from build123d import *

# Parameters (mm, degrees)
F0_R     = 73.025
F1_DEPTH = 3.81
F2_R     = 73.025
F2_R_2   = 69.977
F3_DEPTH = 25.4
F4_R     = 61.2936559159
F5_DEPTH = 25.4
F7_DEPTH = 3.81
F8_W     = 59.7810531035
F8_H     = 29.3873213232
F8_W_2   = 61.7938893847
F9_DEPTH = 127


with BuildPart() as f1:
    # F0 (on Top) → F1 (new body)
    with BuildSketch(Plane.XY):
        Circle(F0_R)
    extrude(amount=F1_DEPTH)

    # F2 (on face) → F3 (join)
    with BuildSketch(Plane.XY.offset(3.81)):
        Circle(F2_R)
        Circle(F2_R_2, mode=Mode.SUBTRACT)
    extrude(amount=F3_DEPTH)

    # F4 (on face) → F5 (cut)
    with BuildSketch(Plane.XY.offset(3.81)):
        Circle(F4_R)
    extrude(amount=-F5_DEPTH, mode=Mode.SUBTRACT)

    # F6 (on face) → F7 (join, through all)
    with BuildSketch(Plane.XY.offset(3.81)):
        with BuildLine():
            Line((3.1198861543, 65.2156993747), (-3.1198873185, 65.2156993747))
            Line((-3.1198873185, 65.2156993747), (-3.1198873185, 9.1467575412))
            ThreePointArc((-3.1198873185, 9.1467575412), (-6.15e-07, 9.6642056268), (3.1198861543, 9.1467579383))
            Line((3.1198861543, 9.1467579383), (3.1198861543, 65.2156993747))
        make_face()
        with BuildLine():
            ThreePointArc((3.1198861543, 9.1467579383), (-6.15e-07, 9.6642056268), (-3.1198873185, 9.1467575412))
            Line((-3.1198873185, 9.1467575412), (-3.1198873185, 3.8243774325))
            Line((-3.1198873185, 3.8243774325), (3.1198861543, 3.8243774325))
            Line((3.1198861543, 3.8243774325), (3.1198861543, 9.1467579383))
        make_face()
        with BuildLine():
            Line((-3.1198873185, 3.8243774325), (-3.1198873185, 9.1467575412))
            ThreePointArc((-3.1198873185, 9.1467575412), (-6.5614847143, 7.0953357033), (-8.8753032428, 3.8243774325))
            Line((-8.8753032428, 3.8243774325), (-3.1198873185, 3.8243774325))
        make_face()
        with BuildLine():
            ThreePointArc((8.8753032428, 3.8243774325), (6.5614842628, 7.0953361208), (3.1198861543, 9.1467579383))
            Line((3.1198861543, 9.1467579383), (3.1198861543, 3.8243774325))
            Line((3.1198861543, 3.8243774325), (8.8753032428, 3.8243774325))
        make_face()
        with BuildLine():
            Line((-3.1198873185, -2.8179625515), (-3.1198873185, 3.8243774325))
            Line((-3.1198873185, 3.8243774325), (-8.8753032428, 3.8243774325))
            ThreePointArc((-8.8753032428, 3.8243774325), (-9.6493328393, 0.5359534999), (-9.2442391497, -2.8179625515))
            Line((-9.2442391497, -2.8179625515), (-3.1198873185, -2.8179625515))
        make_face()
        with BuildLine():
            ThreePointArc((-9.2442391497, -2.8179625515), (-9.6493328393, 0.5359534999), (-8.8753032428, 3.8243774325))
            Line((-8.8753032428, 3.8243774325), (-63.3035078645, 3.8243774325))
            Line((-63.3035078645, 3.8243774325), (-63.3035078645, -2.8179625515))
            Line((-63.3035078645, -2.8179625515), (-9.2442391497, -2.8179625515))
        make_face()
        with BuildLine():
            Line((8.8753032428, 3.8243774325), (3.1198861543, 3.8243774325))
            Line((3.1198861543, 3.8243774325), (3.1198861543, -2.8179625515))
            Line((3.1198861543, -2.8179625515), (9.2442391497, -2.8179625515))
            ThreePointArc((9.2442391497, -2.8179625515), (9.5586374134, -1.4245424514), (9.6642056268, 0))
            ThreePointArc((9.6642056268, 0), (9.4649254074, 1.952449085), (8.8753032428, 3.8243774325))
        make_face()
        with BuildLine():
            Line((64.1086399555, 3.8243774325), (8.8753032428, 3.8243774325))
            ThreePointArc((8.8753032428, 3.8243774325), (9.4649254074, 1.952449085), (9.6642056268, 0))
            ThreePointArc((9.6642056268, 0), (9.5586374134, -1.4245424514), (9.2442391497, -2.8179625515))
            Line((9.2442391497, -2.8179625515), (64.1086399555, -2.8179625515))
            Line((64.1086399555, -2.8179625515), (64.1086399555, 3.8243774325))
        make_face()
        with BuildLine():
            Line((3.1198861543, -2.8179625515), (-3.1198873185, -2.8179625515))
            Line((-3.1198873185, -2.8179625515), (-3.1198873185, -9.1467575412))
            ThreePointArc((-3.1198873185, -9.1467575412), (-6.15e-07, -9.6642056268), (3.1198861543, -9.1467579383))
            Line((3.1198861543, -9.1467579383), (3.1198861543, -2.8179625515))
        make_face()
        with BuildLine():
            Line((-3.1198873185, -9.1467575412), (-3.1198873185, -2.8179625515))
            Line((-3.1198873185, -2.8179625515), (-9.2442391497, -2.8179625515))
            ThreePointArc((-9.2442391497, -2.8179625515), (-6.9448770569, -6.7205322008), (-3.1198873185, -9.1467575412))
        make_face()
        with BuildLine():
            Line((9.2442391497, -2.8179625515), (3.1198861543, -2.8179625515))
            Line((3.1198861543, -2.8179625515), (3.1198861543, -9.1467579383))
            ThreePointArc((3.1198861543, -9.1467579383), (6.9448766292, -6.7205326428), (9.2442391497, -2.8179625515))
        make_face()
        with BuildLine():
            ThreePointArc((3.1198861543, -9.1467579383), (-6.15e-07, -9.6642056268), (-3.1198873185, -9.1467575412))
            Line((-3.1198873185, -9.1467575412), (-3.1198873185, -64.2092823982))
            Line((-3.1198873185, -64.2092823982), (3.1198861543, -64.2092823982))
            Line((3.1198861543, -64.2092823982), (3.1198861543, -9.1467579383))
        make_face()
    extrude(amount=-F7_DEPTH)

    # F8 (on Front) → F9 (cut, symmetric)
    with BuildSketch(Plane.XZ):
        with Locations((-38.0424889736, 19.1218871623)):
            Rectangle(F8_W, F8_H)
        with Locations((36.8347933982, 19.1218871623)):
            Rectangle(F8_W_2, F8_H)
    extrude(amount=F9_DEPTH, both=True, mode=Mode.SUBTRACT)


solid = f1.part
Here's how the part is built. I have some questions about the finished solid (model axes, mm). A direction names the side the tool comes from. Coordinates: 2 decimals unless noted, no trailing zeros. Write each loop counter-clockwise with the first axis right and the second up, starting at its lowest first coordinate (ties: lowest second). Pieces come first, ordered by that corner, then holes.
Item 1: On a 3-axis mill with a long thin cutter (end or side, diameter ignored), from which of +Z, -Z, +X, -X, +Y, -Y can I reach the whole of each face in a straight line? I mean faces 3 (the flat face through (-3.12, 0, 2)), 4 (the flat face through (15, 1, 3.81)), 5 (the flat face through (-67.933, -22, 17)). Say none if no direction works.
Item 2: I want a section at D-D on x = 20. Write out the boundary of the cut face in (y, z), and give its area (3 significant figures).
Item 3: I want a section at C-C on z = 14.25. Write out the boundary of the cut face in (x, y) (3 decimals), and give its area (3 significant figures).
Item 4: If I drill on line 1 (Y direction, x = 0, z = 12.5) (3 decimals); line 2 (X direction, y = -26.5, z = 2); line 3 (Z direction, x = 25, y = 61), over which ranges is the centre line in solid material (lowest first)?
Item 5: I want a section at B-B on y = 0. Write out the boundary of the cut face in (x, z) (3 decimals).
Item 6: I want a section at A-A on x = 0. Write out the boundary of the cut face in (y, z) (3 decimals), and give its area (3 significant figures).
Item 7: If we mould it in two halves opening along X, with no side actions, what happens to faces 1 (the cylindrical face through (6.6, 7.06, 1.93)), 2 (the flat face through (-1, 71, 29.21))? For each: +X half, -X half, draft (parallel to the pull), parting line (faces both ways), or undercut.
Item 8: Will these pins go through, and if not, where does the flat tip stop? pin 1 (1.5 mm diameter, centred on x = 22.5, z = 4.5, fed in from +Y); pin 2 (6 mm diameter, centred on x = 57.5, y = -27.5, fed in from +Z); pin 3 (1.5 mm diameter, centred on y = -71.5, z = 13.5, fed in from -X).
Findings below:
1. face 3: +Z, -Z
1. face 4: +Z
1. face 5: +Z, +Y, -Y
2. outline: (-70.23, 0) - (-57.94, 0) - (-57.94, 3.81) - (-67.06, 3.81) - (-67.06, 4.43) - (-70.23, 4.43) - close; (-2.82, 0) - (3.82, 0) - (3.82, 3.81) - (-2.82, 3.81) - close; (57.94, 0) - (70.23, 0) - (70.23, 4.43) - (67.06, 4.43) - (67.06, 3.81) - (57.94, 3.81) - close
2. area: 123 mm2
3. outline: (-67.933, -26.791) - (-67.933, -16.789) arc R69.977 cw to (-67.933, 16.789) - (-67.933, 26.791) arc R73.025 ccw to start; (-8.152, -72.569) arc R73.025 ccw to (5.938, -72.783) - (5.938, -69.725) arc R69.977 cw to (-8.152, -69.501) - close; (-8.152, 69.501) arc R69.977 cw to (5.938, 69.725) - (5.938, 72.783) arc R73.025 ccw to (-8.152, 72.569) - close; (67.732, -27.296) arc R73.025 ccw to (67.732, 27.296) - (67.732, 17.584) arc R69.977 cw to (67.732, -17.584) - close
3. area: 365 mm2
4. line 1: y = -73.025 to -69.977, 69.977 to 73.025
4. line 2: x = -68.05 to -55.27, -3.12 to 3.12, 55.27 to 68.05
4. line 3: z = 0 to 3.81
5. outline: (-73.025, 0) - (-3.12, 0) - (-3.12, 3.81) - (-69.977, 3.81) - (-69.977, 29.21) - (-73.025, 29.21) - close; (3.12, 0) - (73.025, 0) - (73.025, 29.21) - (69.977, 29.21) - (69.977, 3.81) - (3.12, 3.81) - close
6. outline: (-73.025, 0) - (-2.818, 0) - (-2.818, 3.81) - (-69.977, 3.81) - (-69.977, 29.21) - (-73.025, 29.21) - close; (3.824, 0) - (73.025, 0) - (73.025, 29.21) - (69.977, 29.21) - (69.977, 3.81) - (3.824, 3.81) - close
6. area: 686 mm2
7. face 1: undercut
7. face 2: draft
8. pin 1: stops at y = 69.71
8. pin 2: stops at z = 3.81
8. pin 3: stops at x = -8.15
